Autodesk Fusion 360 part; units mm, degrees
sketch "Sketch1" plane through (0, 0, 0) normal (0, 0, 1) x (1, 0, 0)
  line L0 (0, 500) -> (0, 0)
  line L1 (0, 0) -> (210, 0)
  line L2 (210, 0) -> (210, 500)
  line L3 (210, 500) -> (0, 500)
  line L4 (210, 0) -> (210, 500)
  line L5 (420, 500) -> (420, 0)
  line L6 (210, 500) -> (420, 500)
  line L7 (420, 0) -> (210, 0)
  point P0 (420, 0)
  dimension "d1" = 210
  dimension "d2" = 500
sketch "Sketch2" plane through (0, 0, 0) normal (0, 0, 1) x (1, 0, 0)
  line L0 (33.711, 456.9389) -> (183.711, 456.9389)
  line L1 (183.711, 456.9389) -> (183.711, 376.9389)
  line L2 (183.711, 376.9389) -> (33.711, 376.9389)
  line L3 (33.711, 376.9389) -> (33.711, 456.9389)
  line L4 (210, 0) -> (210, 500)
  line L5 (236.289, 456.9389) -> (236.289, 376.9389)
  line L6 (236.289, 376.9389) -> (386.289, 376.9389)
  line L7 (386.289, 456.9389) -> (236.289, 456.9389)
  line L8 (386.289, 376.9389) -> (386.289, 456.9389)
  dimension "d5" = 80
  dimension "d6" = 150
sketch "Sketch3" plane through (0, 0, 0) normal (0, 0, 1) x (1, 0, 0)
  line L0 (32.2529, 55.6107) -> (182.2529, 55.6107)
  line L1 (182.2529, 55.6107) -> (182.2529, 135.6107)
  line L2 (182.2529, 135.6107) -> (32.2529, 135.6107)
  line L3 (32.2529, 135.6107) -> (32.2529, 55.6107)
  line L4 (210, 0) -> (210, 500)
  line L5 (237.7471, 55.6107) -> (237.7471, 135.6107)
  line L6 (387.7471, 135.6107) -> (387.7471, 55.6107)
  line L7 (237.7471, 135.6107) -> (387.7471, 135.6107)
  line L8 (387.7471, 55.6107) -> (237.7471, 55.6107)
  dimension "d3" = 80
  dimension "d4" = 150
sketch "Sketch4" plane through (0, 0, 0) normal (0, 0, 1) x (1, 0, 0)
  spline S0 degree 5 poles (37.1063, 332.6897) (42.3749, 335.3073) (52.3549, 339.9904) (65.6542, 345.3585) (80.2569, 349.3524) (94.455, 349.9181) (106.0588, 347.1834) (116.552, 342.4363) (127.2275, 337.0505) (138.9022, 332.4525) (151.9574, 330.0384) (163.6176, 330.8449) (173.049, 333.408) (179.6386, 336.0413) (183.0089, 337.5891) knots 0 0 0 0 0 0 0.1 0.2 0.3 0.4 0.5 0.6 0.7 0.8 0.9 1 1 1 1 1 1
  line L0 (12.8551, 320.6405) -> (61.3576, 344.7389)
  spline S1 degree 5 poles (37.1063, 285.0878) (42.8971, 288.4586) (53.8131, 294.4211) (68.19, 301.0281) (83.6155, 305.4358) (98.026, 305.1198) (109.2899, 300.9209) (119.1641, 294.9006) (129.1906, 289.0058) (140.3665, 284.7869) (153.15, 283.3608) (164.7942, 285.1007) (174.3242, 288.2578) (181.0276, 291.2129) (184.4668, 292.9031) knots 0 0 0 0 0 0 0.1 0.2 0.3 0.4 0.5 0.6 0.7 0.8 0.9 1 1 1 1 1 1
  line L1 (11.3971, 270.1228) -> (62.8155, 300.0529)
  line L2 (183.0089, 337.5891) -> (184.4668, 292.9031)
  line L3 (37.1063, 332.6897) -> (37.1063, 285.0878)
  spline S2 degree 5 poles (33.001, 177.9329) (38.3874, 175.2566) (48.5839, 170.5407) (62.1501, 165.3764) (77.0074, 162.0547) (91.4293, 162.4372) (103.2499, 165.5685) (114.0265, 169.6123) (125.0886, 172.9374) (137.2166, 174.4629) (150.704, 173.6089) (162.6105, 170.7864) (172.1303, 167.4148) (178.7303, 164.6061) (182.0937, 163.0615) knots 0 0 0 0 0 0 0.1 0.2 0.3 0.4 0.5 0.6 0.7 0.8 0.9 1 1 1 1 1 1
  line L4 (165.4289, 329.5156) -> (200.5889, 345.6626)
  line L5 (8.7497, 189.9821) -> (57.2522, 165.8837)
  line L6 (164.5136, 171.135) -> (199.6737, 154.988)
  line L7 (33.001, 177.9329) -> (33.001, 225.5347)
  spline S3 degree 5 poles (33.001, 225.5347) (38.5243, 222.3196) (48.8936, 216.5629) (62.4155, 209.9478) (76.6735, 204.9492) (89.8078, 203.8525) (100.2443, 206.3287) (109.9563, 210.6694) (120.5592, 215.2082) (132.869, 218.4944) (147.0982, 219.3055) (159.9368, 217.1832) (170.2893, 213.7191) (177.4957, 210.5385) (181.175, 208.7303) knots 0 0 0 0 0 0 0.1 0.2 0.3 0.4 0.5 0.6 0.7 0.8 0.9 1 1 1 1 1 1
  line L8 (166.2067, 283.9293) -> (202.727, 301.8769)
  line L9 (7.2917, 240.4998) -> (58.7102, 210.5696)
  line L10 (162.9149, 217.7041) -> (199.4352, 199.7565)
  line L11 (182.0937, 163.0615) -> (181.175, 208.7303)
  line L12 (210, 0) -> (210, 500)
  spline S4 degree 5 poles (382.8937, 332.6897) (377.6251, 335.3073) (367.6451, 339.9904) (354.3458, 345.3585) (339.7431, 349.3524) (325.545, 349.9181) (313.9412, 347.1834) (303.448, 342.4363) (292.7725, 337.0505) (281.0978, 332.4525) (268.0426, 330.0384) (256.3824, 330.8449) (246.951, 333.408) (240.3614, 336.0413) (236.9911, 337.5891) knots 0 0 0 0 0 0 0.1 0.2 0.3 0.4 0.5 0.6 0.7 0.8 0.9 1 1 1 1 1 1
  line L13 (407.1449, 320.6405) -> (358.6424, 344.7389)
  line L14 (254.5711, 329.5156) -> (219.4111, 345.6626)
  line L15 (382.8937, 332.6897) -> (382.8937, 285.0878)
  line L16 (237.9063, 163.0615) -> (238.825, 208.7303)
  line L17 (236.9911, 337.5891) -> (235.5332, 292.9031)
  spline S5 degree 5 poles (386.999, 177.9329) (381.6126, 175.2566) (371.4161, 170.5407) (357.8499, 165.3764) (342.9926, 162.0547) (328.5707, 162.4372) (316.7501, 165.5685) (305.9735, 169.6123) (294.9114, 172.9374) (282.7834, 174.4629) (269.296, 173.6089) (257.3895, 170.7864) (247.8697, 167.4148) (241.2697, 164.6061) (237.9063, 163.0615) knots 0 0 0 0 0 0 0.1 0.2 0.3 0.4 0.5 0.6 0.7 0.8 0.9 1 1 1 1 1 1
  line L18 (411.2503, 189.9821) -> (362.7478, 165.8837)
  line L19 (255.4864, 171.135) -> (220.3263, 154.988)
  spline S6 degree 5 poles (386.999, 225.5347) (381.4757, 222.3196) (371.1064, 216.5629) (357.5845, 209.9478) (343.3265, 204.9492) (330.1922, 203.8525) (319.7557, 206.3287) (310.0437, 210.6694) (299.4408, 215.2082) (287.131, 218.4944) (272.9018, 219.3055) (260.0632, 217.1832) (249.7107, 213.7191) (242.5043, 210.5385) (238.825, 208.7303) knots 0 0 0 0 0 0 0.1 0.2 0.3 0.4 0.5 0.6 0.7 0.8 0.9 1 1 1 1 1 1
  line L20 (412.7083, 240.4998) -> (361.2898, 210.5696)
  line L21 (257.0851, 217.7041) -> (220.5648, 199.7565)
  spline S7 degree 5 poles (382.8937, 285.0878) (377.1029, 288.4586) (366.1869, 294.4211) (351.81, 301.0281) (336.3845, 305.4358) (321.974, 305.1198) (310.7101, 300.9209) (300.8359, 294.9006) (290.8094, 289.0058) (279.6335, 284.7869) (266.85, 283.3608) (255.2058, 285.1007) (245.6758, 288.2578) (238.9724, 291.2129) (235.5332, 292.9031) knots 0 0 0 0 0 0 0.1 0.2 0.3 0.4 0.5 0.6 0.7 0.8 0.9 1 1 1 1 1 1
  line L22 (408.6029, 270.1228) -> (357.1845, 300.0529)
  line L23 (253.7933, 283.9293) -> (217.273, 301.8769)
  line L24 (386.999, 177.9329) -> (386.999, 225.5347)
  point P0 (120.393, 340.4922)
  point P1 (123.6058, 292.4233)
  point P2 (117.8255, 170.5984)
  point P3 (112.0744, 211.5163)
  point P4 (307.9256, 211.5163)
  point P5 (299.607, 340.4922)
  point P6 (302.1745, 170.5984)
  point P7 (296.3942, 292.4233)
sketch "Sketch5" plane through (0, 0, 0) normal (0, 0, 1) x (1, 0, 0)
  line L0 (36.9414, 334.4826) -> (36.9414, 288.2338)
sketch "Sketch6" plane through (0, 0, 0) normal (0, 0, 1) x (1, 0, 0)
  line L0 (182.7332, 343.5551) -> (182.7332, 300.0101)
  line L1 (210, 0) -> (210, 500)
  line L2 (237.2668, 343.5551) -> (237.2668, 300.0101)
extrude "Extrude1" add sketch "Sketch1" along normal blind 8 contours L0 L1 L2 L3 L4
extrude "Extrude2" cut sketch "Sketch4" along normal blind 50 contours S2 L7 S3 L11
extrude "Extrude3" cut sketch "Sketch3" along normal blind 50 contours L0 L1 L2 L3
extrude "Extrude4" cut sketch "Sketch2" along normal blind 50 contours L0 L1 L2 L3
extrude "Extrude5" cut sketch "Sketch4" along normal blind 20 contours S0 S1 L2 L3
Verification items for the finished model (mm, model axes). Give positions to 0.01 mm unless a question says otherwise; leave off trailing zeros. Loops run counter-clockwise (first coordinate to the right, second up) from the corner with the lowest first, then second, coordinate; pieces in that order, holes last.
1) Depth check by flat-ended pin: pin 1 Ø4 at (x, z) = (126.5, 2) entering from -Y. Enter the tip coordinate at first touch or a pass-through.
2) Sectioned sample at A-A, the plane y = 88.5. Enter the section's corners in (x, z).
3) Sectioned sample at B-B, the plane z = 2.25. Count the separate pieces of the cut face and the enclosed holes in it, then the cut area to 3 significant figures.
4) Thickness scan on line 1 along Y through (x, z) = (78, 6.75); line 2 along Y through (x, z) = (166, 1.5); line 3 along X through (y, z) = (440, 2.5). Record the ranges inside material, lowest first.
Answers:
1. pin 1: stops at y = 0
2. outline: (0, 0) - (32.25, 0) - (32.25, 8) - (0, 8) - close; (182.25, 0) - (210, 0) - (210, 8) - (182.25, 8) - close
3. separate pieces: 1
3. enclosed holes: 4
3. area: 67,700 mm2
4. line 1: y = 0 to 55.61, 135.61 to 162.97, 205.68 to 303.11, 348.02 to 376.94, 456.94 to 500
4. line 2: y = 0 to 55.61, 135.61 to 169.36, 214.88 to 286, 331.94 to 376.94, 456.94 to 500
4. line 3: x = 0 to 33.71, 183.71 to 210
